Verification items for the finished model (mm, model axes). A direction names the side the tool comes from. Round coordinates to 2 decimals unless told otherwise and drop trailing zeros. Write each loop counter-clockwise with the first axis right and the second up, starting at its lowest first coordinate (ties: lowest second). Pieces come first, ordered by that corner, then holes. Notation, with made-up numbers: (7, -17.5) - (31, -17.5) arc R18 ccw to (31, 12.5) - close; hole circle Ø11 at (71.25, 27). An arc over 180 degrees is marked (long way). Answer as a JSON object with one key per item and string values.
```python
from build123d import *

# Parameters (mm, degrees)
F0_W     = 80.089839
F0_H     = 75.850955
F1_DEPTH = 40
F2_R     = 28.784991
F3_DEPTH = 30
F4_R     = 31.401524
F4_R_2   = 28.550589
F5_DEPTH = 11.5


with BuildPart() as f1:
    # F0 (on Top) → F1 (new body)
    with BuildSketch(Plane.XY):
        with Locations((-9.407865, -16.568296)):
            Rectangle(F0_W, F0_H)
    extrude(amount=F1_DEPTH)

    # F2 (on Top) → F3 (cut)
    with BuildSketch(Plane.XY):
        with Locations((-7.680858, -21.122221)):
            Circle(F2_R)
    extrude(amount=F3_DEPTH, mode=Mode.SUBTRACT)

    # F4 (on face) → F5 (join)
    with BuildSketch(Plane(origin=(0, 0, 0), x_dir=(1, 0, 0), z_dir=(0, 0, -1))):
        with Locations((-7.680858, 21.122221)):
            Circle(F4_R)
        with Locations((-7.680858, 21.122221)):
            Circle(F4_R_2, mode=Mode.SUBTRACT)
    extrude(amount=F5_DEPTH)


solid = f1.part
```
1. Cross-section at D-D (y = 16.5). Record the boundary of the cut face in (x, z).
Completed:
{"outline": "(-49.45, 0) - (30.64, 0) - (30.64, 40) - (-49.45, 40) - close"}
2. Go/stop test with flat-tipped pins: pin 1 (6 mm diameter, centred on y = -1, z = -3.5, fed in from -X); pin 2 (4 mm diameter, centred on y = -32.5, z = -2.5, fed in from -X). Record where each tip stops, or that it passes through.
Completed:
{"pin 1": "stops at x = -34", "pin 2": "stops at x = -37.65"}
3. Cross-section at C-C (z = 28.5). Record the boundary of the cut face in (x, y) (3 decimals), plus the area to 3 significant figures.
Completed:
{"outline": "(-49.453, -54.494) - (30.637, -54.494) - (30.637, 21.357) - (-49.453, 21.357) - close; hole circle Ø57.57 at (-7.681, -21.122)", "area": "3,470 mm^2"}
4. Mould release check, pull along Z, two halves, no side actions. Record for faces 3 (the face through (-1, 7, -11.5)), 4 (the face through (-10, -54.494, 20)), 5 (the face through (-11.428, 7.418, 14.79)), 6 (the face through (-10, -16, 40)): released by +Z, released by -Z, zero draft, split by the parting line, or undercut.
Completed:
{"face 3": "released by -Z", "face 4": "zero draft", "face 5": "undercut", "face 6": "released by +Z"}
5. Material ranges on probe 1 along Y at (x, z) = (-4, 25); probe 2 along Z at (x, y) = (-30, -16); probe 3 along Y at (x, z) = (5.5, 7.5), recorded low to high. Write a range as from..to.
Completed:
{"probe 1": "y = -54.49..-49.67, 7.43..21.36", "probe 2": "z = 30..40", "probe 3": "y = -54.49..-46.71, 4.47..21.36"}
6. Cross-section at B-B (y = -31.5). Record the boundary of the cut face in (x, z).
Completed:
{"outline": "(-49.45, 0) - (-37.32, 0) - (-37.32, -11.5) - (-34.28, -11.5) - (-34.28, 0) - (-34.53, 0) - (-34.53, 30) - (19.17, 30) - (19.17, 0) - (18.92, 0) - (18.92, -11.5) - (21.96, -11.5) - (21.96, 0) - (30.64, 0) - (30.64, 40) - (-49.45, 40) - close"}
7. Access from +Z, -Z, +X, -X, +Y, -Y to the whole of each face (thin tool, end or side, straight path). Record for faces 1 (the face through (-19, 9, 0)), 2 (the face through (-10, 21.357, 20)).
Completed:
{"face 1": "-Z", "face 2": "+Z, -Z, +X, -X, +Y"}
8. Cross-section at A-A (x = 19). Record the boundary of the cut face in (y, z).
Completed:
{"outline": "(-54.49, 0) - (-37.68, 0) - (-37.68, -11.5) - (-31.28, -11.5) - (-31.28, 0) - (-31.93, 0) - (-31.93, 30) - (-10.32, 30) - (-10.32, 0) - (-10.96, 0) - (-10.96, -11.5) - (-4.56, -11.5) - (-4.56, 0) - (21.36, 0) - (21.36, 40) - (-54.49, 40) - close"}
